Answer from the drawing. Dimensions are ordinates in mm from the lowest x, y and z of the part. Round coordinates to 2 decimals unless told otherwise and drop trailing zeros. Order: outer loops, then holes, each group sorted by start corner. A loop starts at its lowest first (then second) coordinate and runs counter-clockwise, first axis right, second up. Notation, with made-up numbers: (87.5, -25.75) -> (135.5, -25.75) arc R26 cw to (135.5, 7.25) -> close; hole circle Ø5 at (-24, 74.25). An arc over 180 degrees is marked (long way). Use a Markdown table: item, result. Add a question column.
Item 1: Find the intervals of material crossed by L1, parallel to Y at x = 33, z = 2.35; L2, parallel to X at y = 54, z = 2.65; L3, parallel to X at y = 68, z = 2.95, in increasing order. Write a range as [from, to].
Item 2: A cutting plane is placed at A-A, the plane y = 50. Determine the outline of the cut face in (x, z) (3 decimals), plus the area to 3 significant figures.
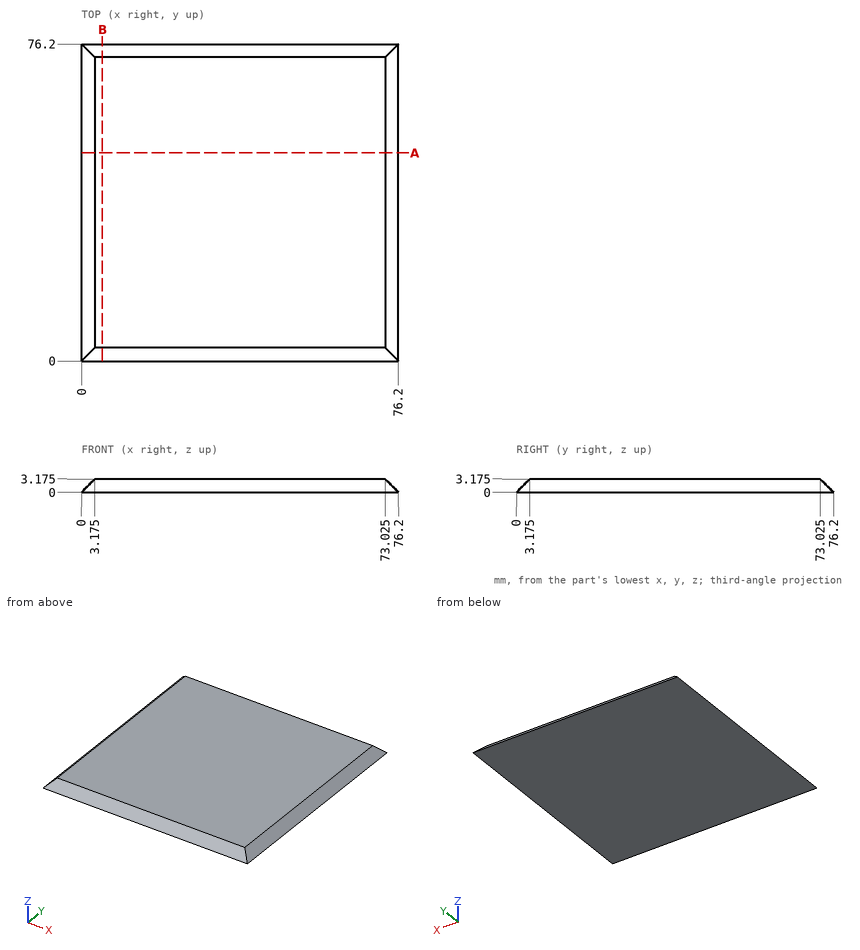
Reported:
| question | item | result |
|---|---|---|
| 1 | L1 | [2.35, 73.85] |
| 1 | L2 | [2.65, 73.55] |
| 1 | L3 | [2.95, 73.25] |
| 2 | outline | (0, 0) -> (76.2, 0) -> (73.025, 3.175) -> (3.175, 3.175) -> close |
| 2 | area | 232 mm² |
